Geometry: see drawing. Coordinates: mm, zero at the bounding-box minimum. Coordinates: 2 decimals unless noted, no trailing zeros. Order: outer loops, then holes, each group sorted by start corner. A loop starts at its lowest first (then second) coordinate and runs counter-clockwise, first axis right, second up.
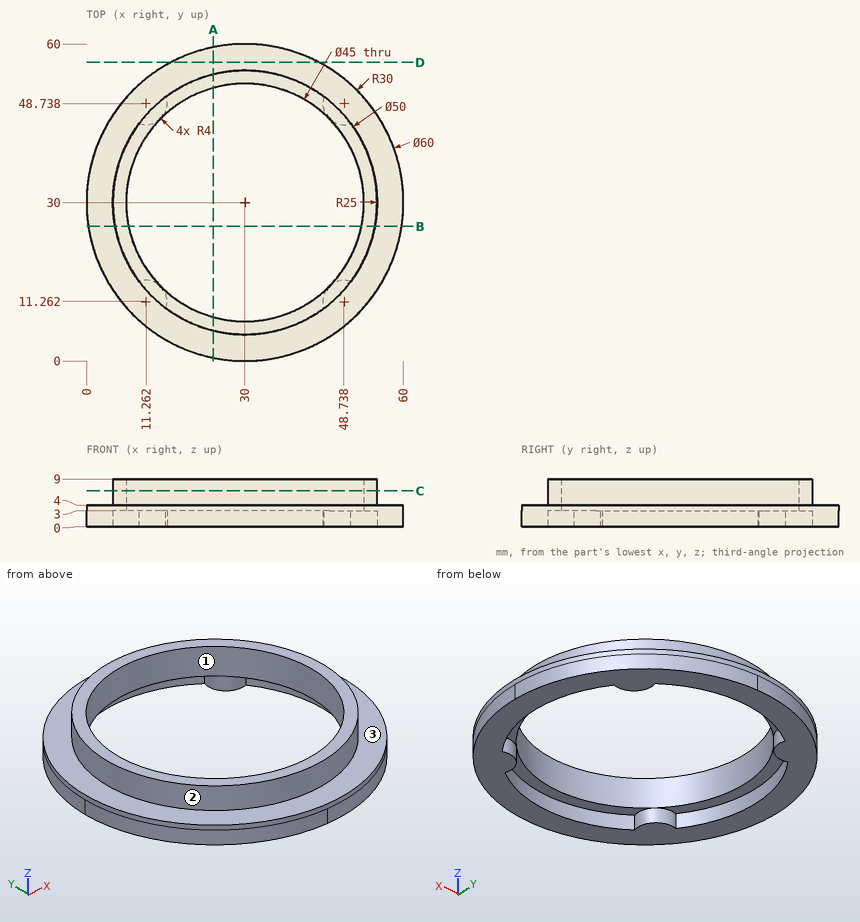
Q1. Section query C-C on z = 6.75. Output: boundary loops of the cut face in (x, y), plus the area to 3 significant figures.
Solutions:
outline: circle Ø50 at (30, 30); hole circle Ø45 at (30, 30)
area: 373 mm2
Q2. Material intervals for line 1 along Y through (x, z) = (30, 5.75); line 2 along Y through (x, z) = (20, 4.5) (1 decimal); line 3 along Z through (x, y) = (7, 37.5), sorted ascending.
Solutions:
line 1: y = 5 to 7.5, 52.5 to 55
line 2: y = 7.1 to 9.8, 50.2 to 52.9
line 3: z = 3 to 9
Q3. Section query A-A on x = 24. Output: boundary loops of the cut face in (y, z) (1 decimal).
Solutions:
outline: (0.6, 0) - (5.7, 0) - (5.7, 3) - (8.3, 3) - (8.3, 9) - (5.7, 9) - (5.7, 4) - (0.6, 4) - close; (51.7, 3) - (54.3, 3) - (54.3, 0) - (59.4, 0) - (59.4, 4) - (54.3, 4) - (54.3, 9) - (51.7, 9) - close
Q4. Pin query (flat end, axial travel): P1, Ø1, axis at x = 8.5, z = 5, coming from the +Y side (1 decimal); P2, Ø7.5, axis at x = 10.5, y = 26.5, coming from the -Z side; P3, Ø3, axis at x = 23, z = 4.5, coming from the +Y side (1 decimal). Return the tip coordinate at first contact, or that it passes through.
Solutions:
P1: stops at y = 43.6
P2: stops at z = 3
P3: stops at y = 59.5
Q5. Pull-direction query (X, two-part tool) for the marked faces 1, 2 and 3; classes: pulls with the +X half, pulls with the -X half, needs draft (parallel to the pull), parting line crosses it, or undercut.
Solutions:
face 1: undercut
face 2: parting line crosses it
face 3: needs draft
Q6. Section query B-B on y = 25.5. Output: boundary loops of the cut face in (x, z) (1 decimal).
Solutions:
outline: (0.3, 0) - (5.4, 0) - (5.4, 3) - (8, 3) - (8, 9) - (5.4, 9) - (5.4, 4) - (0.3, 4) - close; (52, 3) - (54.6, 3) - (54.6, 0) - (59.7, 0) - (59.7, 4) - (54.6, 4) - (54.6, 9) - (52, 9) - close
Q7. Section query D-D on y = 56.5. Output: boundary loops of the cut face in (x, z), plus the area to 4 significant figures.
Solutions:
outline: (15.94, 0) - (44.06, 0) - (44.06, 4) - (15.94, 4) - close
area: 112.5 mm2
